Check sheet for the modelled part. Datum: model origin and axes. Units: mm. Face numbers are marked on the shaded views. A direction names the side the tool comes from. Round coordinates to 2 decimals unless told otherwise and drop trailing zeros. Order: outer loops, then holes, each group sorted by start corner. A loop starts at its lowest first (then second) coordinate and runs counter-clockwise, first axis right, second up.
Q1. Cross-section at D-D on z = 56. Record the cut outline in (x, y).
Q2. Set-up check for the marked faces 5, 6 and 7: record each of +Z, -Z, +X, -X, +Y, -Y from which the full face is reachable in a straight line by a thin tool's end or side.
Q3. Mould release check, pull along Z, two halves, no side actions. Record for the marked faces 1, 2, 3 and 4: +Z half, -Z half, draft (parallel to the pull), parting line (faces both ways), or undercut.
Q4. Depth check by flat-ended pin: P1, Ø7, axis at y = -21, z = 55, coming from the -X side; P2, Ø2, axis at y = 9, z = -12, coming from the +X side; P3, Ø1, axis at x = -4, y = 11, coming from the -Z side; P4, Ø13.5, axis at x = -18.5, z = 27.5, coming from the +Y side. Enter the tip coordinate at first touch or a pass-through.
Q5. Cross-section at B-B on z = 0. Record the cut outline in (x, y), then the cut area to 3 significant figures.
Q6. Scan lines: probe 1 along X at (y, z) = (20, 44.5); probe 2 along Y at (x, z) = (-1, 58); probe 3 along Z at (x, y) = (3.5, -32). Record each from-to range of solid material in increasing order.
Q7. Cross-section at A-A on y = 0. Record the cut outline in (x, z), then the cut area to 3 significant figures.
Q8. Cross-section at C-C on x = -4. Record the cut outline in (y, z), then the cut area to 3 significant figures.
Solid Edge part; units mm, degrees
sketch "Sketch1" plane through (0, 0, 0) normal (0, -1, 0) x (1, 0, 0)
  circle A0 centre (0, 0) radius 30
  circle A1 centre (0, 0) radius 15
extrude "Protrusion1" add sketch "Sketch1" along normal mid plane 80
sketch "Sketch2" plane through (0, 0, 0) normal (0, -1, 0) x (1, 0, 0)
  line L0 (0, 66) -> (40, 66)
  line L1 (40, 66) -> (40, 46)
  line L2 (40, 46) -> (20, 46)
  line L3 (20, 46) -> (20, 33)
  line L4 (20, 33) -> (20, 22.3607)
  line L5 (0, 30) -> (0, 66)
  arc A0 (0, 30) -> (20, 22.3607) centre (0, 0) cw
extrude "ExtrudedProtrusion_2" add sketch "Sketch2" along normal mid plane 60
sketch "Sketch3" plane through (20, 0, 66) normal (0, 0, 1) x (1, 0, 0)
  line L0 (20, 30) -> (20, -30)
  arc A0 (20, 30) -> (20, -30) centre (20, 0) cw
extrude "Protrusion2" add sketch "Sketch3" against normal up to vertex (20 mm away)
sketch "Sketch4" plane through (20, 0, 66) normal (0, 0, 1) x (1, 0, 0)
  circle A0 centre (20, 0) radius 30
extrude "ExtrudedProtrusion_4" add sketch "Sketch4" along normal blind 40
sketch "Sketch5" plane through (40, 0, 106) normal (0, 0, 1) x (1, 0, 0)
  circle A0 centre (0, 0) radius 10
extrude "Cutout1" cut sketch "Sketch5" against normal up to vertex (60 mm away)
sketch "Sketch6" plane through (0, 0, 0) normal (0, -1, 0) x (1, 0, 0)
  line L0 (10, 66) -> (20, 106)
  line L1 (20, 106) -> (10, 106)
  line L2 (10, 106) -> (10, 66)
revolve "RevolvedCutout1" cut sketch "Sketch6" angle 360 about axis through (40, 0, 106) along (0, 0, -1)
sketch "Sketch7" plane through (0, 0, 0) normal (0, -1, 0) x (1, 0, 0)
  arc A0 (-26.7217, 13.6364) -> (0, 30) centre (0, 0) cw
  line L0 (0, 66) -> (-26.7217, 13.6364)
  line L1 (0, 66) -> (0, 30)
extrude "ExtrudedProtrusion_5" add sketch "Sketch7" along normal mid plane 12
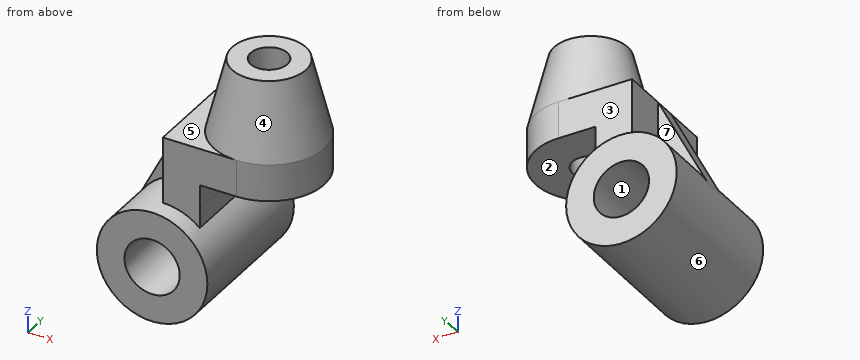
Results found:
1. outline: (-5.1, -6) - (0, -6) - (0, -30) - (40, -30) arc R30 ccw to (40, 30) - (0, 30) - (0, 6) - (-5.1, 6) - close; hole circle Ø20 at (40, 0)
2. face 5: +Z, -X
2. face 6: none
2. face 7: +Z, -X, +Y
3. face 1: undercut
3. face 2: undercut
3. face 3: draft
3. face 4: +Z half
4. P1: stops at x = 0
4. P2: stops at x = 27.91
4. P3: stops at z = -29.8
4. P4: stops at y = 40
5. outline: (-30, -40) - (-15, -40) - (-15, 40) - (-30, 40) - close; (15, -40) - (30, -40) - (30, 40) - (15, 40) - close
5. area: 2,400 mm2
6. probe 1: x = 0 to 20
6. probe 2: y = -6 to 6
6. probe 3: z = -29.8 to -14.59, 14.59 to 29.8
7. outline: (-26.72, 13.64) arc R30 ccw (long way) to (20, 22.36) - (20, 33) - (20, 46) - (30, 46) - (30, 106) - (20, 106) - (10, 66) - (0, 66) - close; (50, 46) - (70, 46) - (70, 66) - (60, 106) - (50, 106) - close; hole circle Ø30 at (0, 0)
7. area: 5,080 mm2
8. outline: (-40, -29.73) - (40, -29.73) - (40, -14.46) - (-40, -14.46) - close; (-40, 14.46) - (40, 14.46) - (40, 29.73) - (6, 29.73) - (6, 58.16) - (-6, 58.16) - (-6, 29.73) - (-40, 29.73) - close
8. area: 2,790 mm2
